Can you work these out from the model? Positions are in its coordinate system, mm. Face numbers are marked on the shaded views. A direction names the side the tool comes from. Give positions to 0.01 mm unless a question says otherwise; leave off trailing zeros.
from build123d import *

# Parameters (mm, degrees)
SKETCH1_R           = 31.75
BOSS_EXTRUDE1_DEPTH = 38.1
FILLET1_R           = 3.175
SKETCH2_R           = 14.2875
CUT_EXTRUDE1_DEPTH  = 19.05
SKETCH3_R           = 4.7625
CUT_EXTRUDE2_DEPTH  = 3.175
SKETCH4_R           = 3.175
CUT_EXTRUDE3_DEPTH  = 51.100654936
CUT_EXTRUDE4_START  = -15.875
SKETCH5_R           = 14.2875
CUT_EXTRUDE4_DEPTH  = 15.875
SKETCH6_R           = 4.7625
BOSS_EXTRUDE2_DEPTH = 9.525
DRAFT2_ANGLE        = 3
SKETCH7_R           = 1.5875
CUT_EXTRUDE5_DEPTH  = 55.99261314


with BuildPart() as part:
    # Sketch1 → Boss-Extrude1 (new body)
    with BuildSketch(Plane(origin=(0, 0, 0), x_dir=(1, 0, 0), z_dir=(0, 1, 0))):
        with Locations(Location((0, 0, 0), (0, 0, 90))):
            Circle(SKETCH1_R)
    extrude(amount=BOSS_EXTRUDE1_DEPTH)

    # Fillet1
    fillet1_edges = [part.edges().sort_by_distance(p)[0] for p in [
        (0, 0, 31.75),
        (0, 38.1, 31.75),
    ]]
    fillet(fillet1_edges, radius=FILLET1_R)

    # Sketch2 → Cut-Extrude1 (cut)
    with BuildSketch(Plane(origin=(0, 38.1, 0), x_dir=(1, 0, 0), z_dir=(0, 1, 0))):
        with Locations(Location((0, 0, 0), (0, 0, 270))):
            Circle(SKETCH2_R)
    extrude(amount=-CUT_EXTRUDE1_DEPTH, mode=Mode.SUBTRACT)

    # Sketch3 → Cut-Extrude2 (cut)
    with BuildSketch(Plane(origin=(0, 19.05, 0), x_dir=(1, 0, 0), z_dir=(0, 1, 0))):
        with Locations(Location((0, 0, 0), (0, 0, 270))):
            Circle(SKETCH3_R)
    extrude(amount=-CUT_EXTRUDE2_DEPTH, mode=Mode.SUBTRACT)

    # Sketch4 → Cut-Extrude3 (cut, through all)
    with BuildSketch(Plane(origin=(0, 15.875, 0), x_dir=(1, 0, 0), z_dir=(0, 1, 0))):
        with Locations(Location((0, 0, 0), (0, 0, 270))):
            Circle(SKETCH4_R)
    extrude(amount=-CUT_EXTRUDE3_DEPTH, mode=Mode.SUBTRACT)

    # Sketch5 → Cut-Extrude4 (cut)
    with BuildSketch(Plane.XZ.offset(CUT_EXTRUDE4_START)):
        with Locations(Location((0, 0, 0), (0, 0, 90))):
            Circle(SKETCH5_R)
    extrude(amount=CUT_EXTRUDE4_DEPTH, mode=Mode.SUBTRACT)

    # Sketch6 → Boss-Extrude2 (add)
    with BuildSketch(Plane(origin=(0, 15.875, 0), x_dir=(-1, 0, 0), z_dir=(0, -1, 0))):
        with BuildLine():
            Line((-9.525, -1), (-6.270765504, -1))
            ThreePointArc((-6.270765504, -1), (-4.978895322, -3.941205573), (-2.412791109, -5.87375))
            ThreePointArc((-2.412791109, -5.87375), (0, -11.1125), (2.412791109, -5.87375))
            ThreePointArc((2.412791109, -5.87375), (4.978895322, -3.941205573), (6.270765504, -1))
            Line((6.270765504, -1), (9.525, -1))
            ThreePointArc((9.525, -1), (10.525, 0), (9.525, 1))
            Line((9.525, 1), (6.270765504, 1))
            ThreePointArc((6.270765504, 1), (4.978895322, 3.941205573), (2.412791109, 5.87375))
            ThreePointArc((2.412791109, 5.87375), (0, 11.1125), (-2.412791109, 5.87375))
            ThreePointArc((-2.412791109, 5.87375), (-4.978895322, 3.941205573), (-6.270765504, 1))
            Line((-6.270765504, 1), (-9.525, 1))
            ThreePointArc((-9.525, 1), (-10.525, 0), (-9.525, -1))
        make_face()
        with Locations(Location((0, 0, 0), (0, 0, 270))):
            Circle(SKETCH6_R, mode=Mode.SUBTRACT)
    extrude(amount=BOSS_EXTRUDE2_DEPTH)

    # Draft2
    draft2_faces = [part.faces().sort_by_distance(p)[0] for p in [
        (10.525, 11.1125, 0),
        (4.978895322, 11.1125, 3.941205573),
        (7.897882752, 11.1125, 1),
        (7.897882752, 11.1125, -1),
        (4.978895322, 11.1125, -3.941205573),
        (0, 11.1125, -11.1125),
        (-7.897882752, 11.1125, 1),
        (-7.897882752, 11.1125, -1),
        (-10.525, 11.1125, 0),
        (-4.978895322, 11.1125, -3.941205573),
        (-4.978895322, 11.1125, 3.941205573),
        (0, 11.1125, 11.1125),
    ]]
    draft(draft2_faces, Plane(origin=(0, 6.35, 0), x_dir=(0, 0, -1), z_dir=(0, -1, 0)), DRAFT2_ANGLE)

    # Sketch7 → Cut-Extrude5 (cut, through all)
    with BuildSketch(Plane(origin=(0, 6.35, 0), x_dir=(-1, 0, 0), z_dir=(0, -1, 0))):
        with Locations(Location((0, 7.9375, 0), (0, 0, 90))):
            Circle(SKETCH7_R)
        with Locations(Location((0, -7.9375, 0), (0, 0, 270))):
            Circle(SKETCH7_R)
    extrude(amount=-CUT_EXTRUDE5_DEPTH, mode=Mode.SUBTRACT)


solid = part.part
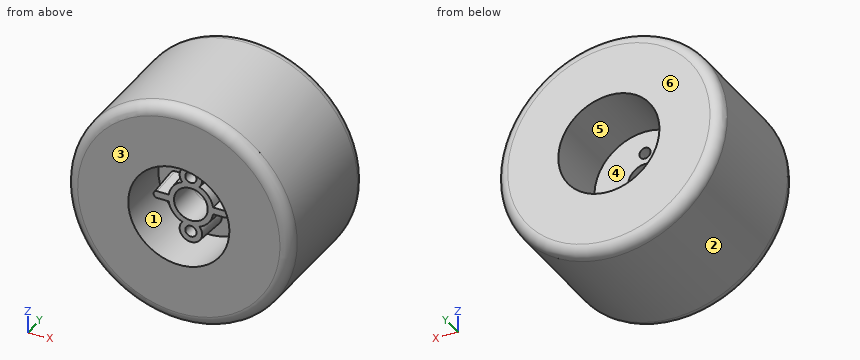
(1) If I drill on L1, parallel to X at y = 23.25, z = 0; L2, parallel to X at y = 10.5, z = 0; L3, parallel to X at y = 18.2, z = 0, over which ranges is the centre line in solid material (lowest first)?
Returned:
L1: x = -31.75 to -14.29, 14.29 to 31.75
L2: x = -31.75 to -14.29, -10.74 to -4.76, 4.76 to 10.74, 14.29 to 31.75
L3: x = -31.75 to -4.76, 4.76 to 31.75
(2) If we mould it in two halves opening along X, with no side actions, what happens to the marked faces 1, 2, 3 and 4? For each: +X half, -X half, draft (parallel to the pull), parting line (faces both ways), or undercut.
Returned:
face 1: undercut
face 2: parting line
face 3: draft
face 4: undercut
(3) Will these pins go through, and if not, where does the flat tip stop? P1, Ø23, axis at x = 0, z = 0, coming from the +Y side; P2, Ø6.5, axis at x = -3, z = 4.5, coming from the -Y side; P3, Ø5, axis at y = 22, z = 6.5, coming from the -X side.
Returned:
P1: stops at y = 19.05
P2: stops at y = 6.35
P3: stops at x = -31.5
(4) Imagine slicing it at B-B, the plane x = 0. Give the number of separate pieces and of enclosed holes in the cut face, plus the area to 3 significant figures.
Returned:
separate pieces: 4
enclosed holes: 0
area: 1,430 mm2
(5) For the marked faces 5 and 6, which set-ups out of +Z, -Z, +X, -X, +Y, -Y let a thin tool reach every point of the face, with its end or its side?
Returned:
face 5: +Y
face 6: +Z, -Z, +X, -X, +Y
